from build123d import *

# Parameters (mm, degrees)
BASE_EXTRUSION_DEPTH = 5
ESQUISSE2_R          = 10
BOSS_EXTRU_1_DEPTH   = 150


with BuildPart() as part:
    # Esquisse1 → Base-Extrusion (new body)
    with BuildSketch(Plane.XY):
        with BuildLine():
            Line((-5, 30.999354832), (-5, 35.999354832))
            Line((-5, 35.999354832), (5, 35.999354832))
            Line((5, 35.999354832), (5, 30.999354832))
            ThreePointArc((5, 30.999354832), (0, -31.4), (-5, 30.999354832))
        make_face()
    extrude(amount=BASE_EXTRUSION_DEPTH)

    # Esquisse2 → Boss.-Extru.1 (add)
    with BuildSketch(Plane(origin=(0, 0, 0), x_dir=(-1, 0, 0), z_dir=(0, 0, -1))):
        Circle(ESQUISSE2_R)
    extrude(amount=BOSS_EXTRU_1_DEPTH)


solid = part.part
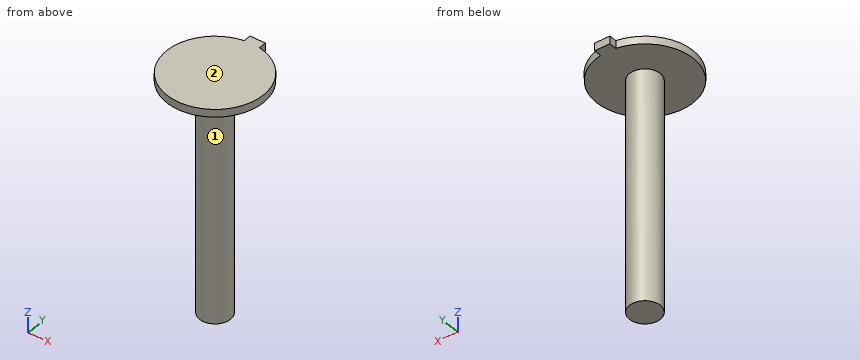
Input: part model. Units: mm. Frame: model coordinates. Face numbers are marked on the shaded views. A direction names the side the tool comes from. Round coordinates to 2 decimals unless told otherwise and drop trailing zeros. Order: outer loops, then holes, each group sorted by start corner. A loop starts at its lowest first (then second) coordinate and runs counter-clockwise, first axis right, second up. Notation, with made-up numbers: (33.25, 39.25) - (69.25, 39.25) arc R9 ccw to (69.25, 43.25) - close; hole circle Ø8 at (80, 37). An arc over 180 degrees is marked (long way). Answer as a JSON object with one key per item and string values. Group by question number.
(1) Pin query (flat end, axial travel): P1, Ø1.5, axis at y = 33, z = 3, coming from the +X side; P2, Ø10, axis at x = 5, z = -33, coming from the +Y side; P3, Ø12, axis at y = 3, z = -41.5, coming from the +X side. Return the tip coordinate at first contact, or that it passes through.
(2) Cut plane D-D (y = -25). Return loops of the section in (x, z), then the cut area to 3 significant figures.
(3) Reachability of the marked faces 1 and 2 from +Z, -Z, +X, -X, +Y, -Y: full face, straight path, thin tool, end or side. Return the list, or none.
(4) Cut plane C-C (z = -134.5). Return loops of the section in (x, y).
(5) Material intervals for probe 1 along Z at (x, y) = (-13, -11); probe 2 along X at (y, z) = (3.5, -50); probe 3 along Y at (x, z) = (7, -142.5), sorted ascending. Write a range as from..to.
(6) Cut plane A-A (x = 0). Return loops of the section in (y, z).
(7) Cut plane B-B (y = 0). Return loops of the section in (x, z), then the cut area to 3 significant figures.
Here are the results:
{
 "1": {"P1": "stops at x = 5", "P2": "stops at y = 10", "P3": "stops at x = 10"},
 "2": {"outline": "(-19, 0) - (19, 0) - (19, 5) - (-19, 5) - close", "area": "190 mm^2"},
 "3": {"face 1": "-Z", "face 2": "+Z, +X, -X, +Y, -Y"},
 "4": {"outline": "circle Ø20 at (0, 0)"},
 "5": {"probe 1": "z = 0..5", "probe 2": "x = -9.37..9.37", "probe 3": "y = -7.14..7.14"},
 "6": {"outline": "(-31.4, 0) - (-10, 0) - (-10, -150) - (10, -150) - (10, 0) - (36, 0) - (36, 5) - (-31.4, 5) - close"},
 "7": {"outline": "(-31.4, 0) - (-10, 0) - (-10, -150) - (10, -150) - (10, 0) - (31.4, 0) - (31.4, 5) - (-31.4, 5) - close", "area": "3,310 mm^2"}
}
